from build123d import *


with BuildPart() as f1:
    # F0 (on Top) → F1 (revolve)
    with BuildSketch(Plane.XY):
        Polygon((-12.367387, 3.325909), (0, 3.002057), (0, 12), (-15.092844, 12), (-15.092844, 3.397277), align=None)
        Polygon((0, 3.002057), (0, 2.5), (16.290502, 2.5), (16.290502, 12), (0, 12), align=None)
    revolve(axis=Axis((-6.948064, 0.181941, 0), (-0.999657, 0.026177, 0)))


solid = f1.part
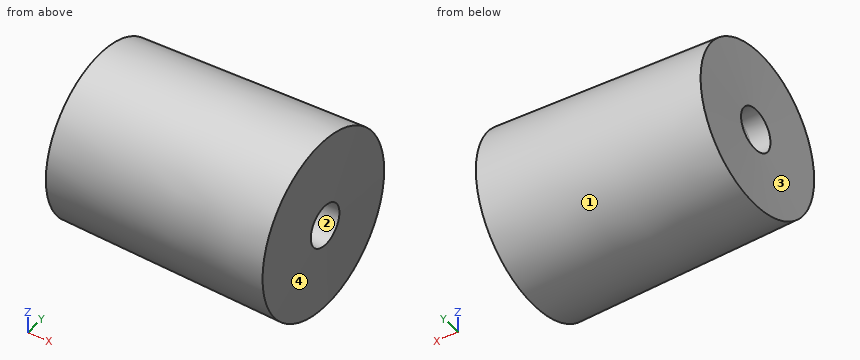
Could you check a few things on this model? Use its own coordinates, in mm. Face numbers are marked on the shaded views. A direction names the side the tool comes from. Coordinates: 2 decimals unless noted, no trailing zeros. One line per question, with ' | ' between items.
Q1. I'm going to push flat-ended pins straight in: P1, Ø1.5, axis at y = -7.5, z = 3.5, coming from the +X side; P2, Ø12, axis at x = 6.5, y = 5.5, coming from the -Z side; P3, Ø1.5, axis at x = 2, z = 6, coming from the +Y side. Where does each tip first touch, or does it pass through?
Return value:
P1: x = 15.94 | P2: z = -12.24 | P3: y = 10.8
Q2. If I drill on L1, parallel to Y at x = -14, z = 0; L2, parallel to X at y = 10, z = -0.75; L3, parallel to Z at x = -12, y = 1.75, over which ranges is the centre line in solid material (lowest first)?
Return value:
L1: -11.28 to -2.64, 3.37 to 12 | L2: -15.09 to 16.29 | L3: -11.6 to -2.64, 2.64 to 11.6
Q3. On a 3-axis mill with a long thin cutter (end or side, diameter ignored), from which of +Z, -Z, +X, -X, +Y, -Y can I reach the whole of each face in a straight line? I mean the marked faces 3 and 4. Say none if no direction works.
Return value:
face 3: -X, +Y | face 4: +X, -Y
Q4. Thinking about a two-plate mould opening in Y: for the marked faces 1 and 2, which applies, pulls with the +Y half, pulls with the -Y half, needs draft (parallel to the pull), parting line crosses it, or undercut?
Return value:
face 1: parting line crosses it | face 2: undercut
